```python
from build123d import *

# Parameters (mm, degrees)
SKETCH2_R                 = 3.9751
BOSS_EXTRUDE1_DEPTH       = 17.2
M4X0_7_TAPPED_HOLE1_D     = 3.3
M4X0_7_TAPPED_HOLE1_DEPTH = 10
M4X0_7_TAPPED_HOLE1_TIP   = 0.991420021
M4X0_7_TAPPED_HOLE2_D     = 3.3
M4X0_7_TAPPED_HOLE2_DEPTH = 10
M4X0_7_TAPPED_HOLE2_TIP   = 0.991420021


with BuildPart() as part:
    # Sketch2 → Boss-Extrude1 (new body, symmetric)
    with BuildSketch(Plane(origin=(0, 0, 0), x_dir=(1, 0, 0), z_dir=(0, 1, 0))):
        Circle(SKETCH2_R)
    extrude(amount=BOSS_EXTRUDE1_DEPTH, both=True)

    # M4x0.7 Tapped Hole1
    with Locations(Plane(origin=(0, 17.2, 0), x_dir=(1, 0, 0), z_dir=(0, 1, 0))):
        with Locations((0, 0)):
            Hole(M4X0_7_TAPPED_HOLE1_D / 2, depth=M4X0_7_TAPPED_HOLE1_DEPTH)
            with Locations((0, 0, -(M4X0_7_TAPPED_HOLE1_DEPTH + M4X0_7_TAPPED_HOLE1_TIP / 2))):  # 118° drill point
                Cone(0, M4X0_7_TAPPED_HOLE1_D / 2, M4X0_7_TAPPED_HOLE1_TIP, mode=Mode.SUBTRACT)

    # M4x0.7 Tapped Hole2
    with Locations(Plane(origin=(0, -17.2, 0), x_dir=(-1, 0, 0), z_dir=(0, -1, 0))):
        with Locations((0, 0)):
            Hole(M4X0_7_TAPPED_HOLE2_D / 2, depth=M4X0_7_TAPPED_HOLE2_DEPTH)
            with Locations((0, 0, -(M4X0_7_TAPPED_HOLE2_DEPTH + M4X0_7_TAPPED_HOLE2_TIP / 2))):  # 118° drill point
                Cone(0, M4X0_7_TAPPED_HOLE2_D / 2, M4X0_7_TAPPED_HOLE2_TIP, mode=Mode.SUBTRACT)


solid = part.part
```
Geometry: final body of the model. Coordinates: model frame, mm. A direction names the side the tool comes from. Give positions to 0.01 mm unless a question says otherwise; leave off trailing zeros. Loops run counter-clockwise (first coordinate to the right, second up) from the corner with the lowest first, then second, coordinate; pieces in that order, holes last. Notation, with made-up numbers: (6, 22.5) -> (10, 22.5) arc R28 ccw to (10, 51.5) -> close; hole circle Ø1 at (59, 32). An arc over 180 degrees is marked (long way). Use one line per item in the form item = value.
Item 1: Line query: probe 1 along Z at (x, y) = (0, 15.5); probe 2 along X at (y, z) = (10, -0.25); probe 3 along Z at (x, y) = (-1.5, -14.5). Output: solid intervals per line, ascending.
A:
probe_1 = -3.98 to -1.65, 1.65 to 3.98
probe_2 = -3.97 to -1.63, 1.63 to 3.97
probe_3 = -3.68 to -0.69, 0.69 to 3.68
Item 2: Section query C-C on x = 3.5. Output: boundary loops of the cut face in (y, z), and give its area (3 significant figures).
A:
outline = (-17.2, -1.88) -> (17.2, -1.88) -> (17.2, 1.88) -> (-17.2, 1.88) -> close
area = 130 mm^2
Item 3: Section query D-D on x = 2. Output: boundary loops of the cut face in (y, z).
A:
outline = (-17.2, -3.44) -> (17.2, -3.44) -> (17.2, 3.44) -> (-17.2, 3.44) -> close
Item 4: Draft query along X for faces 1 (the face through (2, 17.2, 0)), 2 (the face through (-0.86, 0.24, 3.88)), 3 (the face through (0.3, 6.4, 0.1)). Return one class per face: pulls with the +X half, pulls with the -X half, needs draft (parallel to the pull), parting line crosses it, or undercut.
A:
face_1 = needs draft
face_2 = parting line crosses it
face_3 = undercut
Item 5: Access query for faces 4 (the face through (-1.216, -12.13, -1.115)), 5 (the face through (2, -17.2, 0)), 6 (the face through (1.216, 12.13, -1.115)). Directions: +Z, -Z, +X, -X, +Y, -Y. A direction counts if a zero-diameter tool reaches every point of the face in a straight line with its end or side. Return the directions, or none.
A:
face_4 = -Y
face_5 = +Z, -Z, +X, -X, -Y
face_6 = +Y
Item 6: Pin query (flat end, axial travel): P1, Ø2.5, axis at x = 0, z = 0, coming from the -Y side; P2, Ø2, axis at x = 2.5, y = 4, coming from the +Z side. Return the tip coordinate at first contact, or that it passes through.
A:
P1 = -6.96
P2 = 3.68
Item 7: Section query B-B on y = -4. Output: boundary loops of the cut face in (x, z).
A:
outline = circle Ø7.95 at (0, 0)
Item 8: Section query A-A on y = 8. Output: boundary loops of the cut face in (x, z).
A:
outline = circle Ø7.95 at (0, 0); hole circle Ø3.3 at (0, 0)
